Autodesk Inventor part; units mm, degrees
ref_plane "YZ Plane" through (0, 0, 0) normal (1, 0, 0) x (0, 1, 0)
ref_plane "XZ Plane" through (0, 0, 0) normal (0, 1, 0) x (-1, 0, 0)
ref_plane "XY Plane" through (0, 0, 0) normal (0, 0, 1) x (1, 0, 0)
sketch "Sketch1" plane through (0, 0, 0) normal (0, 0, 1) x (1, 0, 0)
  line L0 (0, 0) -> (25.4, 0)
  line L1 (25.4, 0) -> (25.4, 50.8)
  line L2 (25.4, 50.8) -> (0, 50.8)
  line L3 (0, 50.8) -> (0, 0)
  line L4 (22.225, 47.625) -> (22.225, 3.175)
  line L5 (22.225, 3.175) -> (3.175, 3.175)
  line L6 (3.175, 3.175) -> (3.175, 47.625)
  line L7 (3.175, 47.625) -> (22.225, 47.625)
  dimension "d0" = 25.4
  dimension "d1" = 50.8
  dimension "d2" = 3.175
extrude "Extrusion1" add sketch "Sketch1" along normal blind 254
sketch "Sketch4" plane through (0, 50.8, 0) normal (0, 1, 0) x (1, 0, 0)
  line L0 (0, -254) -> (25.4, -254)
  line L1 (25.4, 0) -> (25.4, -254)
  line L2 (25.4, 0) -> (0, 0)
  line L3 (0, 0) -> (0, -254)
  line L4 (25.4, -254) -> (-35.2095, -60.0497)
  line L5 (-35.2095, -60.0497) -> (25.4, -41.1092)
  line L6 (25.4, -254) -> (25.4, -41.1092)
  line L7 (0, -49.0467) -> (0, -172.72)
  dimension "d17" = 203.2
  dimension "d18" = 63.5
extrude "Extrusion4" cut sketch "Sketch4" against normal blind 254 contours L3 L4 L0 | L5 L3 L2 L1
properties part number "ball shoot" material "Aluminum 6061"
Verification items for the finished model (mm, model axes). A direction names the side the tool comes from. Give positions to 0.01 mm unless a question says otherwise; leave off trailing zeros. Loops run counter-clockwise (first coordinate to the right, second up) from the corner with the lowest first, then second, coordinate; pieces in that order, holes last. Notation, with made-up numbers: M 16.5,67.5 L 55.5,67.5 A15 cw 55.5,76.5 Z; hole C -32.5,-4 d10. An arc over 180 degrees is marked long. Return JSON: item names as keys, results as strings.
1) Section check A-A, the plane z = 97.5. Enter the section's corners in (x, y) (3 decimals).
Findings:
{"outline": "M 0,0 L 25.4,0 L 25.4,50.8 L 0,50.8 Z; hole M 3.175,3.175 L 22.225,3.175 L 22.225,47.625 L 3.175,47.625 Z"}
2) Section check C-C, the plane x = 11. Enter the section's corners in (y, z) (3 decimals), and give its area (3 significant figures).
Findings:
{"outline": "M 0,45.609 L 3.175,45.609 L 3.175,207.92 L 0,207.92 Z; M 47.625,45.609 L 50.8,45.609 L 50.8,207.92 L 47.625,207.92 Z", "area": "1,030 mm2"}
3) Gauge pin test, flat end, axial feed: P1, Ø6, axis at y = 21.5, z = 209.5, coming from the -X side (3 decimals). Record the tip position at first contact, or that the pin passes through.
Findings:
{"P1": "stops at x = 22.225"}
4) Material ranges on L1, parallel to X at y = 34, z = 102 (3 decimals); L2, parallel to Y at x = 18.25, z = 204 (3 decimals); L3, parallel to X at y = 23.5, z = 226 (3 decimals), recorded low to high. Write a range as [from, to].
Findings:
{"L1": "x = [0, 3.175], [22.225, 25.4]", "L2": "y = [0, 3.175], [47.625, 50.8]", "L3": "x = [22.225, 25.4]"}
5) Section check B-B, the plane y = 13.5. Enter the section's corners in (x, z) (3 decimals), and give its area (3 significant figures).
Findings:
{"outline": "M 0,49.047 L 3.175,48.055 L 3.175,182.88 L 0,172.72 Z; M 22.225,42.101 L 25.4,41.109 L 25.4,254 L 22.225,243.84 Z", "area": "1,070 mm2"}
6) Section check D-D, the plane z = 239. Enter the section's corners in (x, y) (1 decimal), and give its area (3 significant figures).
Findings:
{"outline": "M 20.7,0 L 25.4,0 L 25.4,50.8 L 20.7,50.8 L 20.7,47.6 L 22.2,47.6 L 22.2,3.2 L 20.7,3.2 Z", "area": "171 mm2"}
7) Tool access check on faces 1 (the flat face through (3.175, 25, 115)), 2 (the flat face through (25.4, 25, 146)). Record the directions out of +Z, -Z, +X, -X, +Y, -Y that give a thin tool (end or side, any length) a straight path to the whole face; none if there is none.
Findings:
{"face 1": "+Z, -Z", "face 2": "+Z, -Z, +X, +Y, -Y"}
8) Mould release check, pull along Y, two halves, no side actions. Record for faces 3 (the flat face through (13, 0, 122)), 4 (the flat face through (2.29, 23.64, 48.33)), 5 (the flat face through (22.225, 26, 142)): released by +Y, released by -Y, zero draft, split by the parting line, or undercut.
Findings:
{"face 3": "released by -Y", "face 4": "zero draft", "face 5": "undercut"}
